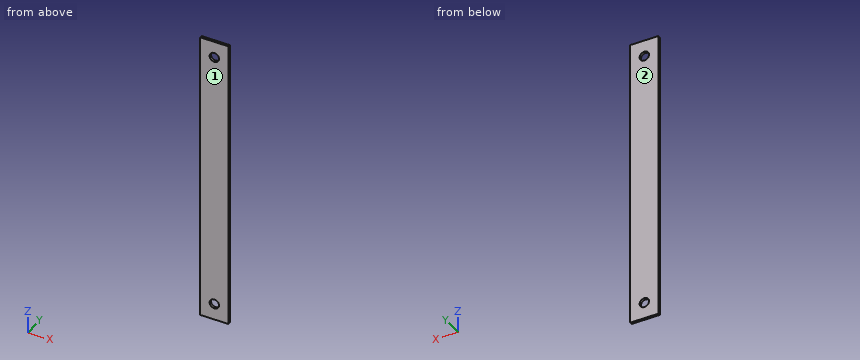
Autodesk Inventor part; units mm, degrees
ref_plane "YZ Plane" through (0, 0, 0) normal (1, 0, 0) x (0, 1, 0)
ref_plane "XZ Plane" through (0, 0, 0) normal (0, 1, 0) x (-1, 0, 0)
ref_plane "XY Plane" through (0, 0, 0) normal (0, 0, 1) x (1, 0, 0)
sketch "Sketch1" plane through (0, 0, 0) normal (0, 1, 0) x (-1, 0, 0)
  line L0 (0, 0) -> (12, 0)
  line L1 (12, 0) -> (12, -125)
  line L2 (12, -125) -> (0, -125)
  line L3 (0, -125) -> (0, 0)
  circle A0 centre (6, -7) radius 2
  circle A1 centre (6, -118) radius 2
  dimension "d0" = 12
  dimension "d1" = 125
  dimension "d2" = 4
  dimension "d6" = 7
  dimension "d7" = 6
  dimension "d36" = 4
  dimension "d37" = 111
  dimension "d38" = 7
extrude "Extrusion1" add sketch "Sketch1" along normal blind 1
sketch "Sketch4" plane through (0, 1, 0) normal (0, 1, 0) x (1, 0, 0)
  circle A0 centre (-6, 118) radius 2
  line L0 (-6, 118) -> (-6, 62.5) construction
  circle A1 centre (-6, 62.5) radius 55.5
  point P0 (0, 0)
  point P1 (-6, 3.7)
  dimension "d39" = 55.5
properties part number "Heater Fixing Bar" material "Aluminum 6061"
Can you work these out from the model? Positions are in its coordinate system, mm. Face numbers are marked on the shaded views. Round coordinates to 2 decimals unless told otherwise and drop trailing zeros. Loops run counter-clockwise (first coordinate to the right, second up) from the corner with the lowest first, then second, coordinate; pieces in that order, holes last. Notation, with made-up numbers: M -37.5,-5 L 8.5,-5 A14 cw 8.5,3 Z; hole C 85,-23.75 d2. An arc over 180 degrees is marked long. Write item = value, one per line. Start each with the question number.
(1) Suppose I cut it at C-C on z = -7. Write out the boundary of the cut face in (x, y), plus the area to 3 significant figures.
(2) I need wall thicknesses on line 1 along Z through (x, y) = (-6, 0.5); line 2 along Z through (x, y) = (-7.75, 0.5); line 3 along X through (y, z) = (0.8, -6.5). Which ranges of each line are inside material? Lowest first, please.
(3) Suppose I cut it at A-A on x = -6. Write out the boundary of the cut face in (y, z), plus the area to 3 significant figures.
(4) I'm going to push a flat-ended pin straight in: P1, Ø3, axis at x = -6, z = -118, coming from the -Y side. Where does the tip first touch, or does it pass through?
(5) If we mould it in two halves opening along Y, with no side actions, what happens to the marked faces 1 and 2? For each: released by +Y, released by -Y, zero draft, split by the parting line, or undercut.
(6) Suppose I cut it at B-B on y = 0.65. Write out the boundary of the cut face in (x, z), plus the area to 3 significant figures.
Answer block:
q1.outline = M -12,0 L -8,0 L -8,1 L -12,1 Z; M -4,0 L 0,0 L 0,1 L -4,1 Z
q1.area = 8.00 mm²
q2.line_1 = -125 to -120, -116 to -9, -5 to 0
q2.line_2 = -125 to -118.97, -117.03 to -7.97, -6.03 to 0
q2.line_3 = -12 to -7.94, -4.06 to 0
q3.outline = M 0,-125 L 1,-125 L 1,-120 L 0,-120 Z; M 0,-116 L 1,-116 L 1,-9 L 0,-9 Z; M 0,-5 L 1,-5 L 1,0 L 0,0 Z
q3.area = 117 mm²
q4.P1 = through
q5.face_1 = released by -Y
q5.face_2 = released by +Y
q6.outline = M -12,-125 L 0,-125 L 0,0 L -12,0 Z; hole C -6,-118 d4; hole C -6,-7 d4
q6.area = 1,470 mm²
